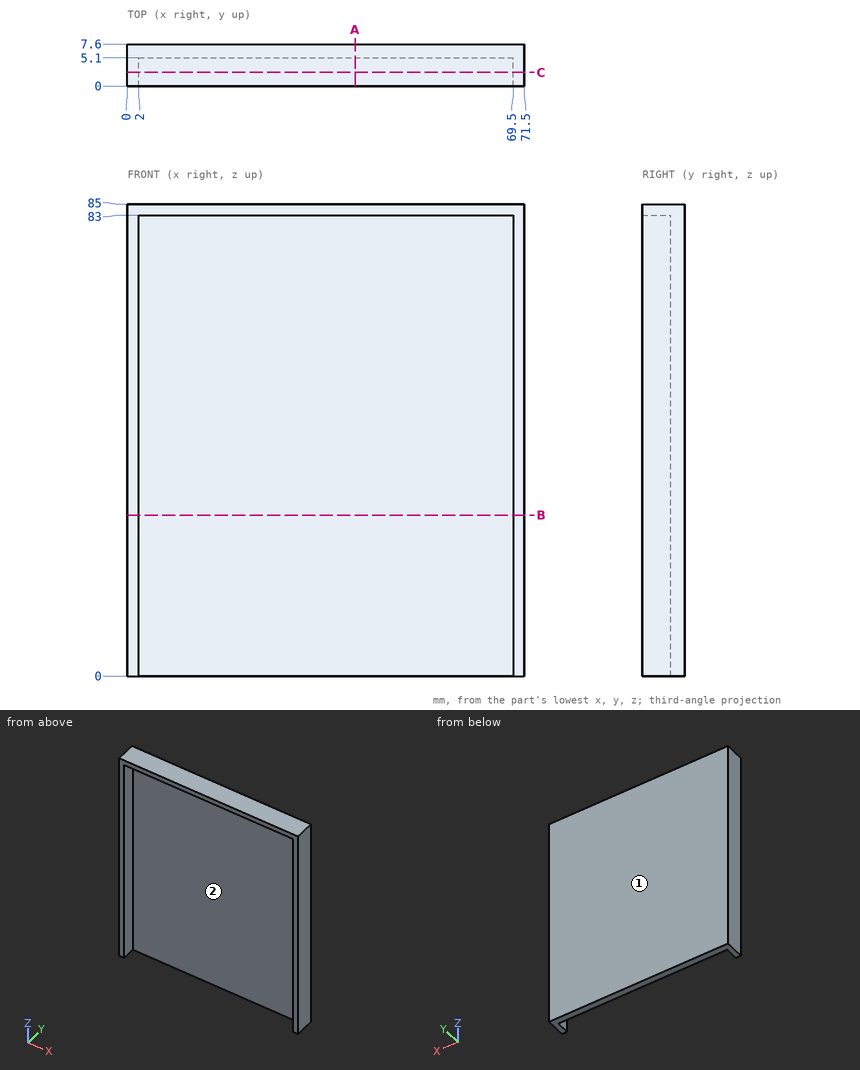
For this review, use the dimensioned drawing (mm, ordinates from the lowest corner) and the shaded views. Round coordinates to 2 decimals unless told otherwise and drop trailing zeros. Order: outer loops, then holes, each group sorted by start corner. A loop starts at its lowest first (then second) coordinate and runs counter-clockwise, first axis right, second up. Notation, with made-up numbers: M 30.25,36 L 60.25,36 A9 cw 60.25,53 Z; hole C 36,10 d5. An arc over 180 degrees is marked long. Use a Markdown table: item, result. Add a question column.
Item 1: Mouldability with a two-part tool opening along X and no side actions: class the marked faces 1 and 2 as released by +X, released by -X, zero draft, split by the parting line, or undercut.
Item 2: Add section C-C, the plane y = 2.5. Give the boundary of the cut face in (x, z).
Item 3: Add section B-B, the plane z = 29. Give the boundary of the cut face in (x, y), then the cut area to 3 significant figures.
Item 4: Insertion check: pin 1 (1 mm diameter, centred on x = 32, y = 4, fed in from -Z); pin 2 (2 mm diameter, centred on y = 3.5, z = 53.5, fed in from -X). Each pin has a flat end and moves straight along its axis. Give the tip position at first contact, or say it passes through.
Item 5: Add section A-A, the plane x = 41. Give the boundary of the cut face in (y, z).
Item 6: To check wall thickness, follow line 1 along X through (y, z) = (3.5, 7); line 2 along Y through (x, z) = (48.5, 56); line 3 along Z through (x, y) = (25.5, 3). State the ranges of each line that lie inside material, in increasing order.
Geometry results:
| question | item | result |
|---|---|---|
| 1 | face 1 | zero draft |
| 1 | face 2 | undercut |
| 2 | outline | M 0,0 L 2,0 L 2,83 L 69.5,83 L 69.5,0 L 71.5,0 L 71.5,85 L 0,85 Z |
| 3 | outline | M 0,0 L 2,0 L 2,5.1 L 69.5,5.1 L 69.5,0 L 71.5,0 L 71.5,7.6 L 0,7.6 Z |
| 3 | area | 199 mm² |
| 4 | pin 1 | stops at z = 83 |
| 4 | pin 2 | stops at x = 0 |
| 5 | outline | M 0,83 L 5.1,83 L 5.1,0 L 7.6,0 L 7.6,85 L 0,85 Z |
| 6 | line 1 | x = 0 to 2, 69.5 to 71.5 |
| 6 | line 2 | y = 5.1 to 7.6 |
| 6 | line 3 | z = 83 to 85 |
